Source: CAD feature listing. Evaluate the final solid. Frame: model axes, mm. Face numbers are marked on the shaded views. A direction names the side the tool comes from. Coordinates: 2 decimals unless noted, no trailing zeros. Write each loop counter-clockwise with the first axis right and the second up, starting at its lowest first coordinate (ties: lowest second). Pieces come first, ordered by that corner, then holes. Notation, with made-up numbers: (-16, 37.25) - (-12, 37.25) arc R25 cw to (-12, 71.25) - close; hole circle Ø11 at (-19.75, -40). An arc over 180 degrees is marked (long way). One line per question, with ' | ' between items.
from build123d import *

# Parameters (mm, degrees)
F0_W     = 50
F0_H     = 50
F1_DEPTH = 30
F2_W     = 30
F2_H     = 5
F2_R     = 15
F3_DEPTH = 30.001
F4_R     = 10
F5_DEPTH = 15


# Not quite as in the source:
# - a pattern or mirror of a feature is missing from the dataset's text; its kind, count and spacing are read off the source's solid


with BuildPart() as f1:
    # F0 (on Right) → F1 (new body)
    with BuildSketch(Plane.YZ):
        Rectangle(F0_W, F0_H)
    extrude(amount=-F1_DEPTH)

    # F2 (on face) → F3 (cut, through all)
    with BuildSketch(Plane.YZ):
        with Locations((0, 22.5)):
            Rectangle(F2_W, F2_H)
        with Locations((0, -25)):
            Circle(F2_R)
    extrude(amount=-F3_DEPTH, mode=Mode.SUBTRACT)

    # F4 (on face) → F5 (join)
    with BuildSketch(Plane(origin=(-30, 0, 0), x_dir=(0, -1, 0), z_dir=(-1, 0, 0))):
        with BuildLine():
            Line((45, 20), (25, 20))
            Line((25, 20), (25, -10))
            Line((25, -10), (45, -10))
            ThreePointArc((45, -10), (55.6066017178, -5.6066017178), (60, 5))
            ThreePointArc((60, 5), (55.6066017178, 15.6066017178), (45, 20))
        make_face()
        with Locations((45, 5)):
            Circle(F4_R, mode=Mode.SUBTRACT)
    f5 = extrude(amount=-F5_DEPTH)

    # F5_copies: F5 across plane
    add(f5.mirror(Plane.ZX))


solid = f1.part
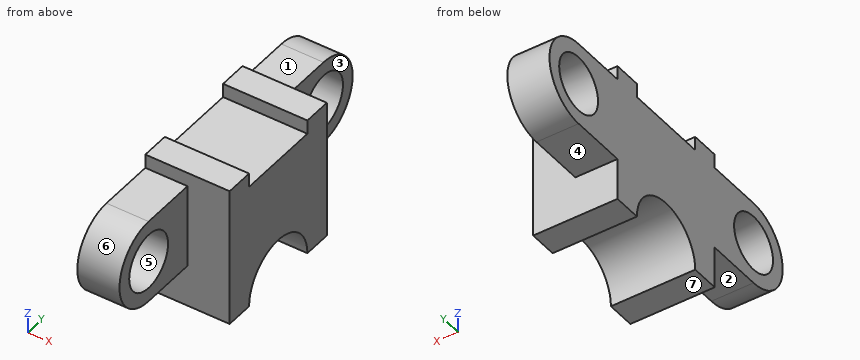
Item 1: Pin query (flat end, axial travel): pin 1 Ø12 at (x, y) = (-20.5, 47.5) entering from -Z; pin 2 Ø3 at (x, y) = (-14, 6) entering from +Z; pin 3 Ø3 at (x, z) = (-6.5, 15) entering from -Y. Return the tip coordinate at first contact, or that it passes through.
Check sheet entries:
pin 1: z = -10 | pin 2: z = 20 | pin 3: y = -25
Item 2: Access query for the marked faces 1, 2, 3 and 4. Directions: +Z, -Z, +X, -X, +Y, -Y. A direction counts if a zero-diameter tool reaches every point of the face in a straight line with its end or side. Return the directions, or none.
Check sheet entries:
face 1: +Z, +X, -X, +Y | face 2: -Z, +X, -X, -Y | face 3: +Z, -Z, +X, +Y | face 4: -Z, +X, -X, +Y
Item 3: Cut plane B-B on x = -21.5. Return loops of the section in (y, z), and give its area (3 significant figures).
Check sheet entries:
outline: (-45, -10) - (-25, -10) - (-25, -25) - (-15, -25) arc R15 cw to (15, -25) - (25, -25) - (25, -10) - (45, -10) arc R15 ccw to (45, 20) - (25, 20) - (25, 25) - (15, 25) - (15, 20) - (-15, 20) - (-15, 25) - (-25, 25) - (-25, 20) - (-45, 20) arc R15 ccw to start; hole circle Ø20 at (-45, 5); hole circle Ø20 at (45, 5) | area: 3,280 mm²
Item 4: Mould query, pull axis Y, two halves, no side actions, for the marked faces 5, 6 and 7. Classes: pulls with the +Y half, pulls with the -Y half, needs draft (parallel to the pull), parting line crosses it, or undercut.
Check sheet entries:
face 5: undercut | face 6: pulls with the -Y half | face 7: needs draft
Item 5: Ray query, line 1 along Z through (x, y) = (-21.75, 45); line 2 along Y through (x, z) = (-25.25, -4); line 3 along Y through (x, z) = (-12.25, 21). Return the intervals inside material, ascending. Write a range as [from, to].
Check sheet entries:
line 1: [-10, -5], [15, 20] | line 2: [-57, -49.36], [-40.64, 40.64], [49.36, 57] | line 3: [-25, -15], [15, 25]
Item 6: Cut plane C-C on x = -6. Return loops of the section in (y, z).
Check sheet entries:
outline: (-25, -25) - (-15, -25) arc R15 cw to (15, -25) - (25, -25) - (25, 25) - (15, 25) - (15, 20) - (-15, 20) - (-15, 25) - (-25, 25) - close
Item 7: Cut plane A-A on z = 5. Return loops of the section in (x, y).
Check sheet entries:
outline: (-30, -60) - (-15, -60) - (-15, -55) - (-30, -55) - close; (-30, -35) - (-15, -35) - (-15, -25) - (0, -25) - (0, 25) - (-15, 25) - (-15, 35) - (-30, 35) - close; (-30, 55) - (-15, 55) - (-15, 60) - (-30, 60) - close
Item 8: Cut plane D-D on z = -12. Return loops of the section in (x, y), and give its area (3 significant figures).
Check sheet entries:
outline: (-30, -25) - (0, -25) - (0, -7.48) - (-30, -7.48) - close; (-30, 7.48) - (0, 7.48) - (0, 25) - (-30, 25) - close | area: 1,050 mm²
